Answer from the drawing. Dimensions are ordinates in mm from the lowest x, y and z of the part. A direction names the side the tool comes from. Give positions to 0.01 mm unless a question says otherwise; leave off trailing zeros. Order: outer loops, then holes, each group sorted by start corner. A loop starts at its lowest first (then second) coordinate and runs counter-clockwise, first axis right, second up. Notation, with made-up numbers: (52.25, 49) - (67.25, 49) arc R25 cw to (67.25, 61) - close; hole circle Ø2 at (18, 81.5). An arc over 180 degrees is marked (long way). Write each question's results on one line, items separated by ' | '.
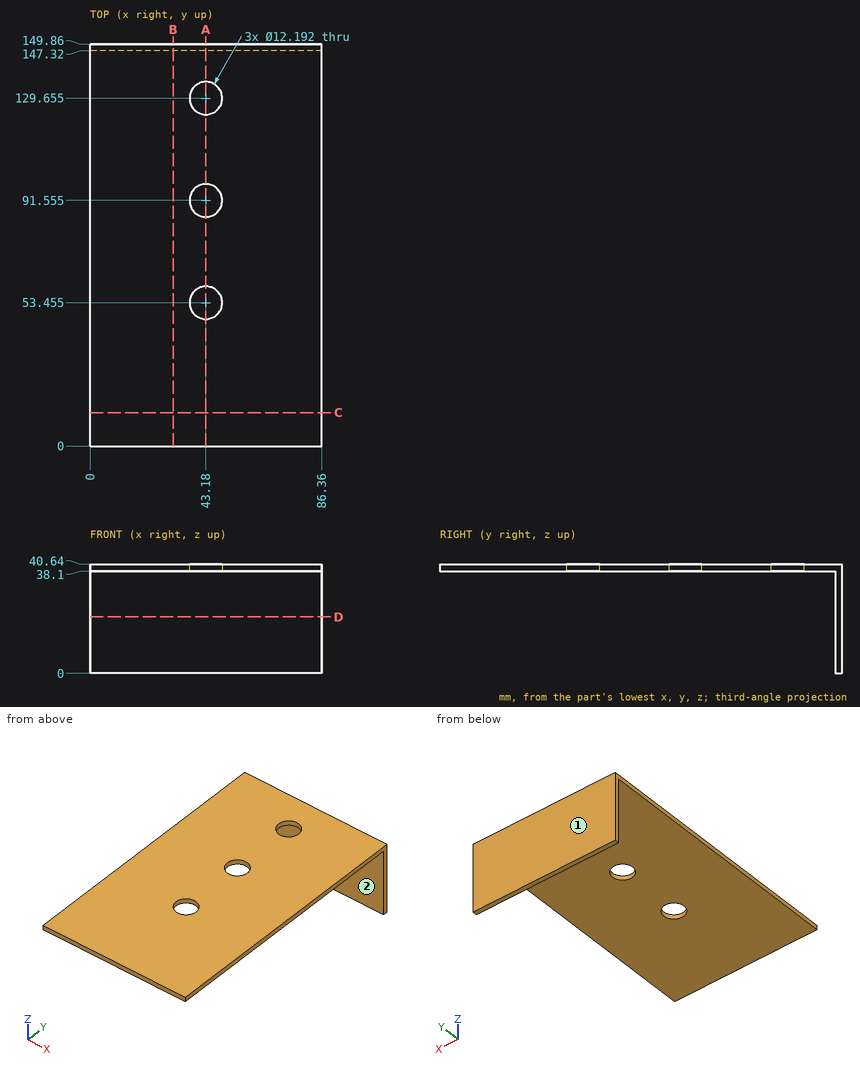
(1) Section A-A (x = 43.18) is taken. Give the vertices of the cut face in (y, z).
Conclusion:
outline: (0, 38.1) - (47.36, 38.1) - (47.36, 40.64) - (0, 40.64) - close; (59.55, 38.1) - (85.46, 38.1) - (85.46, 40.64) - (59.55, 40.64) - close; (97.65, 38.1) - (123.56, 38.1) - (123.56, 40.64) - (97.65, 40.64) - close; (135.75, 38.1) - (147.32, 38.1) - (147.32, 0) - (149.86, 0) - (149.86, 40.64) - (135.75, 40.64) - close
(2) Section C-C (y = 12.5) is taken. Give the vertices of the cut face in (x, z).
Conclusion:
outline: (0, 38.1) - (86.36, 38.1) - (86.36, 40.64) - (0, 40.64) - close
(3) Each of these flat-tipped pins is pushed along its axis until it touches: pin 1 (6 mm diameter, centred on x = 47, y = 104.5, fed in from -Z); pin 2 (2 mm diameter, centred on x = 42.5, z = 7.5, fed in from -Y); pin 3 (1.5 mm diameter, centred on y = 43, z = 35.5, fed in from +X). Where does it stop, or does it pass through?
Conclusion:
pin 1: z = 38.1 | pin 2: y = 147.32 | pin 3: through
(4) Section B-B (x = 31) is taken. Give the vertices of the cut face in (y, z).
Conclusion:
outline: (0, 38.1) - (147.32, 38.1) - (147.32, 0) - (149.86, 0) - (149.86, 40.64) - (0, 40.64) - close
(5) Section D-D (z = 21) is taken. Give the vertices of the cut face in (x, y).
Conclusion:
outline: (0, 147.32) - (86.36, 147.32) - (86.36, 149.86) - (0, 149.86) - close
(6) Consider probe 1 along Y at (x, z) = (43.18, 39.45); probe 2 along Y at (x, z) = (28.5, 10.5); probe 3 along Z at (x, y) = (65, 69). Determine where each line is inside the solid, lowest interval first. Write a range as [from, to].
Conclusion:
probe 1: [0, 47.36], [59.55, 85.46], [97.65, 123.56], [135.75, 149.86] | probe 2: [147.32, 149.86] | probe 3: [38.1, 40.64]
(7) For the marked faces 1 and 2, determine the directions among +Z, -Z, +X, -X, +Y, -Y from which every point of the face is accessible in a straight line to the end or side of a thin tool.
Conclusion:
face 1: +Z, -Z, +X, -X, +Y | face 2: -Z, +X, -X, -Y
